Source: CAD feature listing. Evaluate the final solid. Frame: model axes, mm. Give positions to 0.01 mm unless a question says otherwise; leave off trailing zeros. Order: outer loops, then holes, each group sorted by start corner. A loop starts at its lowest first (then second) coordinate and runs counter-clockwise, first axis right, second up. Notation, with made-up numbers: (-5, -13) -> (48, -13) arc R17 ccw to (48, 17) -> close; hole circle Ø6 at (-23.5, 49). An arc over 180 degrees is marked (long way). Use CSV: the item, a comma, the result in double quotes.
```python
from build123d import *

# Parameters (mm, degrees)
F0_R     = 6.35
F0_R_2   = 19.05
F1_DEPTH = 12.7


# Not quite as in the source:
# - a feature names something its author has since deleted; it is built from what else it names


with BuildPart() as f1:
    # F0 (on Top) → F1 (new body)
    with BuildSketch(Plane.XY):
        with BuildLine():
            ThreePointArc((76.2, 31.75), (70.6203841816, 45.2203841816), (57.15, 50.8))
            Line((57.15, 50.8), (-57.15, 50.8))
            ThreePointArc((-57.15, 50.8), (-70.6203841816, 45.2203841816), (-76.2, 31.75))
            Line((-76.2, 31.75), (-76.2, -31.75))
            ThreePointArc((-76.2, -31.75), (-70.6203841816, -45.2203841816), (-57.15, -50.8))
            Line((-57.15, -50.8), (57.15, -50.8))
            ThreePointArc((57.15, -50.8), (70.6203841816, -45.2203841816), (76.2, -31.75))
            Line((76.2, -31.75), (76.2, 31.75))
        make_face()
        with Locations((-57.15, -31.75)):
            Circle(F0_R, mode=Mode.SUBTRACT)
        with Locations((57.15, -31.75)):
            Circle(F0_R, mode=Mode.SUBTRACT)
        Circle(F0_R_2, mode=Mode.SUBTRACT)
        with Locations((-57.15, 31.75)):
            Circle(F0_R, mode=Mode.SUBTRACT)
        with Locations((57.15, 31.75)):
            Circle(F0_R, mode=Mode.SUBTRACT)
    extrude(amount=F1_DEPTH)


solid = f1.part
```
1. Mould query, pull axis Y, two halves, no side actions, for faces 1 (the flat face through (76.2, 0, 6)), 2 (the cylindrical face through (70.77, 45.07, 6.26)), 3 (the cylindrical face through (-15.12, -11.59, 6.26)), 4 (the cylindrical face through (-62.2, 27.9, 6.3)). Classes: released by +Y, released by -Y, zero draft, split by the parting line, or undercut.
Answer below:
face 1,"zero draft"
face 2,"released by +Y"
face 3,"undercut"
face 4,"undercut"
2. Section query C-C on z = 3. Return loops of the section in (x, y).
Answer below:
outline,"(-76.2, -31.75) arc R19.05 ccw to (-57.15, -50.8) -> (57.15, -50.8) arc R19.05 ccw to (76.2, -31.75) -> (76.2, 31.75) arc R19.05 ccw to (57.15, 50.8) -> (-57.15, 50.8) arc R19.05 ccw to (-76.2, 31.75) -> close; hole circle Ø12.7 at (-57.15, -31.75); hole circle Ø12.7 at (-57.15, 31.75); hole circle Ø38.1 at (0, 0); hole circle Ø12.7 at (57.15, -31.75); hole circle Ø12.7 at (57.15, 31.75)"
3. Ray query, line 1 along Y through (x, z) = (57.15, 9.5); line 2 along Y through (x, z) = (-63, 4.25); line 3 along Y through (x, z) = (0, 7). Return the intervals inside material, ascending.
Answer below:
line 1,"y = -50.8 to -38.1, -25.4 to 25.4, 38.1 to 50.8"
line 2,"y = -49.88 to -34.22, -29.28 to 29.28, 34.22 to 49.88"
line 3,"y = -50.8 to -19.05, 19.05 to 50.8"
4. Section query D-D on y = -28. Return loops of the section in (x, z), plus the area to 3 significant figures.
Answer below:
outline,"(-76.2, 0) -> (-62.27, 0) -> (-62.27, 12.7) -> (-76.2, 12.7) -> close; (-52.03, 0) -> (52.03, 0) -> (52.03, 12.7) -> (-52.03, 12.7) -> close; (62.27, 0) -> (76.2, 0) -> (76.2, 12.7) -> (62.27, 12.7) -> close"
area,"1,680 mm²"
5. Section query B-B on y = -5.5. Return loops of the section in (x, z), plus the area to 3 significant figures.
Answer below:
outline,"(-76.2, 0) -> (-18.24, 0) -> (-18.24, 12.7) -> (-76.2, 12.7) -> close; (18.24, 0) -> (76.2, 0) -> (76.2, 12.7) -> (18.24, 12.7) -> close"
area,"1,470 mm²"
6. Section query A-A on x = 0. Return loops of the section in (y, z), plus the area to 3 significant figures.
Answer below:
outline,"(-50.8, 0) -> (-19.05, 0) -> (-19.05, 12.7) -> (-50.8, 12.7) -> close; (19.05, 0) -> (50.8, 0) -> (50.8, 12.7) -> (19.05, 12.7) -> close"
area,"806 mm²"
